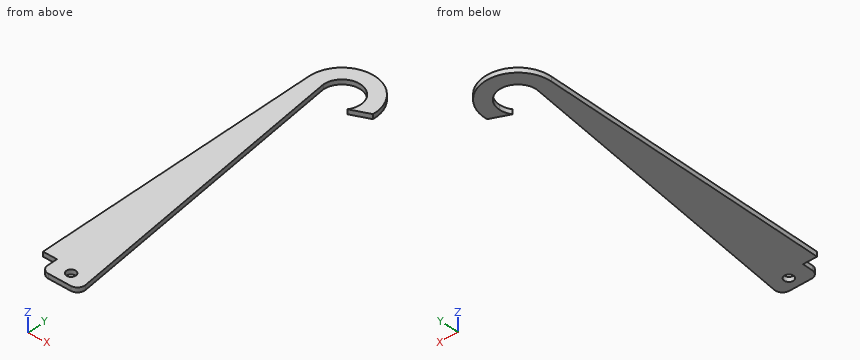
```python
from build123d import *

# Parameters (mm, degrees)
SKETCH1_R           = 6.35
BOSS_EXTRUDE1_DEPTH = 6.35
FILLET1_R           = 10


with BuildPart() as part:
    # Sketch1 → Boss-Extrude1 (new body)
    with BuildSketch(Plane.XY):
        with BuildLine():
            Line((3.331127109, 389.92455355), (27.90992579, 401.162728042))
            ThreePointArc((27.90992579, 401.162728042), (-15.607198263, 450.028916488), (-62.759573024, 404.660447113))
            Line((-62.759573024, 404.660447113), (-62.759573024, 6.090179643))
            Line((-62.759573024, 6.090179643), (-43.715258354, 6.090179643))
            Line((-43.715258354, 6.090179643), (-43.715258354, -17.785820357))
            Line((-43.715258354, -17.785820357), (8.125653236, -17.785820357))
            Line((8.125653236, -17.785820357), (-42.757358599, 404.660447113))
            ThreePointArc((-42.757358599, 404.660447113), (-17.357358599, 430.060447113), (8.042641401, 404.660447113))
            ThreePointArc((8.042641401, 404.660447113), (6.83610681, 396.925058855), (3.331127109, 389.92455355))
        make_face()
        with Locations((-17.357358599, -1.739552887)):
            Circle(SKETCH1_R, mode=Mode.SUBTRACT)
    extrude(amount=BOSS_EXTRUDE1_DEPTH)

    # Fillet1
    fillet1_edges = [part.edges().sort_by_distance(p)[0] for p in [
        (8.125653236, -17.785820357, 3.175),
        (-43.715258354, -17.785820357, 3.175),
    ]]
    fillet(fillet1_edges, radius=FILLET1_R)


solid = part.part
```
Geometry: final body of the model. Coordinates: model frame, mm. Round coordinates to 2 decimals unless told otherwise and drop trailing zeros. Write each loop counter-clockwise with the first axis right and the second up, starting at its lowest first coordinate (ties: lowest second). Pieces come first, ordered by that corner, then holes. Notation, with made-up numbers: M 70,-0.75 L 125,-0.75 A18 cw 125,12.25 Z; hole C 47.25,51 d8. An arc over 180 degrees is marked long. Answer in a Markdown table with one row per item. Add a question column.
(1) Cut plane C-C, the plane y = 321. Return the cut outline in (x, z).
(2) Cut plane B-B, the plane x = 21.5. Return the cut outline in (y, z).
(3) Cut plane A-A, the plane z = 1.25. Return the cut outline in (x, y).
(4) Ray query, L1, parallel to X at y = 401, z = 5.25; L2, parallel to X at y = 329, z = 2.5; L3, parallel to X at y = 176, z = 1.75. Return the intervals inside material, ascending.
(5) Contact query for flat-ended pins moving along their axis: pin 1 (3 mm diameter, centred on x = -21, y = 191.5, fed in from -Z); pin 2 (3 mm diameter, centred on y = 86, z = 1.5, fed in from +X); pin 3 (1 mm diameter, centred on x = -43, z = 2, fed in from +Y); pin 4 (1 mm diameter, centred on y = 87.5, z = 5.5, fed in from +X). Output: stop coordinate, or through.
Established:
| question | item | result |
|---|---|---|
| 1 | outline | M -62.76,0 L -32.68,0 L -32.68,6.35 L -62.76,6.35 Z |
| 2 | outline | M 398.23,0 L 428.14,0 L 428.14,6.35 L 398.23,6.35 Z |
| 3 | outline | M -62.76,6.09 L -43.72,6.09 L -43.72,-7.79 A10 ccw -33.72,-17.79 L -3.15,-17.79 A10 ccw 6.78,-6.59 L -42.76,404.66 A25.4 cw long 3.33,389.92 L 27.91,401.16 A45.4 ccw long -62.76,404.66 Z; hole C -17.36,-1.74 d12.7 |
| 4 | L1 | -62.76 to -42.32, 7.78 to 27.55 |
| 4 | L2 | -62.76 to -33.64 |
| 4 | L3 | -62.76 to -15.22 |
| 5 | pin 1 | z = 0 |
| 5 | pin 2 | x = -4.19 |
| 5 | pin 3 | y = 442.47 |
| 5 | pin 4 | x = -4.5 |
